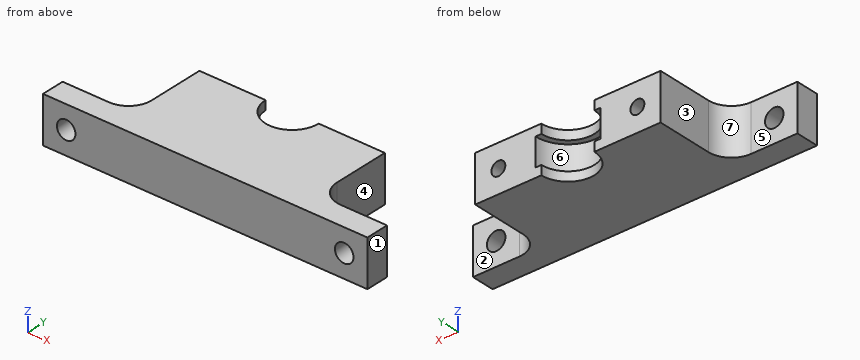
from build123d import *

# Parameters (mm, degrees)
SKETCH1_W           = 40
SKETCH1_H           = 10
BOSS_EXTRUDE1_DEPTH = 22.1798
CUT_EXTRUDE1_DEPTH  = 3
CUT_EXTRUDE2_DEPTH  = 5
SKETCH4_R           = 1.5
CUT_EXTRUDE3_DEPTH  = 7
SKETCH5_W           = 15
SKETCH5_H           = 10
SKETCH5_R           = 2
BOSS_EXTRUDE2_DEPTH = 5
FILLET1_R           = 5


with BuildPart() as part:
    # Sketch1 → Boss-Extrude1 (new body)
    with BuildSketch(Plane(origin=(0, 0, 0), x_dir=(1, 0, 0), z_dir=(0, 1, 0))):
        Rectangle(SKETCH1_W, SKETCH1_H)
    extrude(amount=BOSS_EXTRUDE1_DEPTH)

    # Sketch2 → Cut-Extrude1 (cut, symmetric)
    with BuildSketch(Plane(origin=(0, 0, 0), x_dir=(-1, 0, 0), z_dir=(0, 0, -1))):
        with BuildLine():
            Line((-6.985, 22.1798), (6.985, 22.1798))
            ThreePointArc((6.985, 22.1798), (0, 15.1948), (-6.985, 22.1798))
        make_face()
    extrude(amount=CUT_EXTRUDE1_DEPTH, both=True, mode=Mode.SUBTRACT)

    # Sketch3 → Cut-Extrude2 (cut, symmetric)
    with BuildSketch(Plane(origin=(0, 0, 0), x_dir=(-1, 0, 0), z_dir=(0, 0, -1))):
        with BuildLine():
            Line((-5.715, 22.1798), (5.715, 22.1798))
            ThreePointArc((5.715, 22.1798), (0, 16.4648), (-5.715, 22.1798))
        make_face()
    extrude(amount=CUT_EXTRUDE2_DEPTH, both=True, mode=Mode.SUBTRACT)

    # Sketch4 → Cut-Extrude3 (cut)
    with BuildSketch(Plane(origin=(0, 22.1798, 0), x_dir=(1, 0, 0), z_dir=(0, 1, 0))):
        with Locations((15, 0)):
            Circle(SKETCH4_R)
        with Locations((-15, 0)):
            Circle(SKETCH4_R)
    extrude(amount=-CUT_EXTRUDE3_DEPTH, mode=Mode.SUBTRACT)

    # Sketch5 → Boss-Extrude2 (add)
    with BuildSketch(Plane.XZ):
        with Locations((-27.5, 0)):
            Rectangle(SKETCH5_W, SKETCH5_H)
        with Locations((-30, 0)):
            Circle(SKETCH5_R, mode=Mode.SUBTRACT)
        with Locations((27.5, 0)):
            Rectangle(SKETCH5_W, SKETCH5_H)
        with Locations((30, 0)):
            Circle(SKETCH5_R, mode=Mode.SUBTRACT)
    extrude(amount=-BOSS_EXTRUDE2_DEPTH)

    # Fillet1
    fillet1_edges = [part.edges().sort_by_distance(p)[0] for p in [
        (-20, 5, 0),
        (20, 5, 0),
    ]]
    fillet(fillet1_edges, radius=FILLET1_R)


solid = part.part
Read the model definition and answer for the solid it produces. Units are mm, in the model's axes. Face numbers are marked on the shaded views. A direction names the side the tool comes from. Give positions to 0.01 mm unless a question says otherwise; leave off trailing zeros. Write each loop counter-clockwise with the first axis right and the second up, starting at its lowest first coordinate (ties: lowest second). Pieces come first, ordered by that corner, then holes. Notation, with made-up numbers: (-32.75, 41.5) - (7.25, 41.5) arc R12 ccw to (7.25, 55.5) - close; hole circle Ø10 at (-34.75, -21). An arc over 180 degrees is marked (long way). Answer in a Markdown table with one row per item. Add a question column.
Item 1: Section B-B, the plane y = 4.25 is taken. Write down the section's boundary in (x, z), and give its area (3 significant figures).
Item 2: Determine the mould class of the marked faces 4, 5, 6 and 7 for opening direction X: pulls with the +X half, pulls with the -X half, needs draft (parallel to the pull), parting line crosses it, or undercut.
Item 3: Section A-A, the plane x = -30 is taken. Write down the section's boundary in (y, z), and give its area (3 significant figures).
Item 4: Flat-ended cylindrical pins translate along their axes: P1, Ø5, axis at y = 20, z = -3, coming from the +X side; P2, Ø2, axis at x = 3.5, y = 20, coming from the -Z side; P3, Ø1.5, axis at x = -14.5, z = -0.5, coming from the +Y side; P4, Ø5, axis at x = -27, z = -1.5, coming from the +Y side. Find the tip coordinate at first contact, or state that the pin passes through.
Item 5: Find the intervals of material crossed by L1, parallel to Z at x = -30, y = 3.35; L2, parallel to X at y = 18.5, z = -1; L3, parallel to X at y = 20.25, z = 0, in increasing order.
Item 6: Section D-D, the plane x = 15 is taken. Write down the section's boundary in (y, z), and give its area (3 significant figures).
Item 7: A tool of negligible diameter and unlimited length cuts with its end or side. For the marked faces 1, 2 and 3, from which of +Z, -Z, +X, -X, +Y, -Y can it reach the whole face along a straight path? Write none if from no direction.
Item 8: Section C-C, the plane z = -3.75 is taken. Write down the section's boundary in (x, y) (3 decimals).
Recorded:
| question | item | result |
|---|---|---|
| 1 | outline | (-35, -5) - (35, -5) - (35, 5) - (-35, 5) - close; hole circle Ø4 at (-30, 0); hole circle Ø4 at (30, 0) |
| 1 | area | 675 mm2 |
| 2 | face 4 | pulls with the +X half |
| 2 | face 5 | needs draft |
| 2 | face 6 | undercut |
| 2 | face 7 | pulls with the -X half |
| 3 | outline | (0, -5) - (5, -5) - (5, -2) - (0, -2) - close; (0, 2) - (5, 2) - (5, 5) - (0, 5) - close |
| 3 | area | 30.0 mm2 |
| 4 | P1 | stops at x = 20 |
| 4 | P2 | passes through |
| 4 | P3 | stops at y = 15.18 |
| 4 | P4 | stops at y = 5.03 |
| 5 | L1 | z = -5 to -2, 2 to 5 |
| 5 | L2 | x = -20 to -16.12, -13.88 to -5.94, 5.94 to 13.88, 16.12 to 20 |
| 5 | L3 | x = -20 to -16.5, -13.5 to -6.71, 6.71 to 13.5, 16.5 to 20 |
| 6 | outline | (0, -5) - (22.18, -5) - (22.18, -1.5) - (15.18, -1.5) - (15.18, 1.5) - (22.18, 1.5) - (22.18, 5) - (0, 5) - close |
| 6 | area | 201 mm2 |
| 7 | face 1 | +Z, -Z, +X, +Y, -Y |
| 7 | face 2 | +Z, -Z, +X, +Y |
| 7 | face 3 | +Z, -Z, -X, +Y |
| 8 | outline | (-35, 0) - (35, 0) - (35, 5) - (25, 5) arc R5 cw to (20, 10) - (20, 22.18) - (5.715, 22.18) arc R5.715 cw to (-5.715, 22.18) - (-20, 22.18) - (-20, 10) arc R5 cw to (-25, 5) - (-35, 5) - close |
